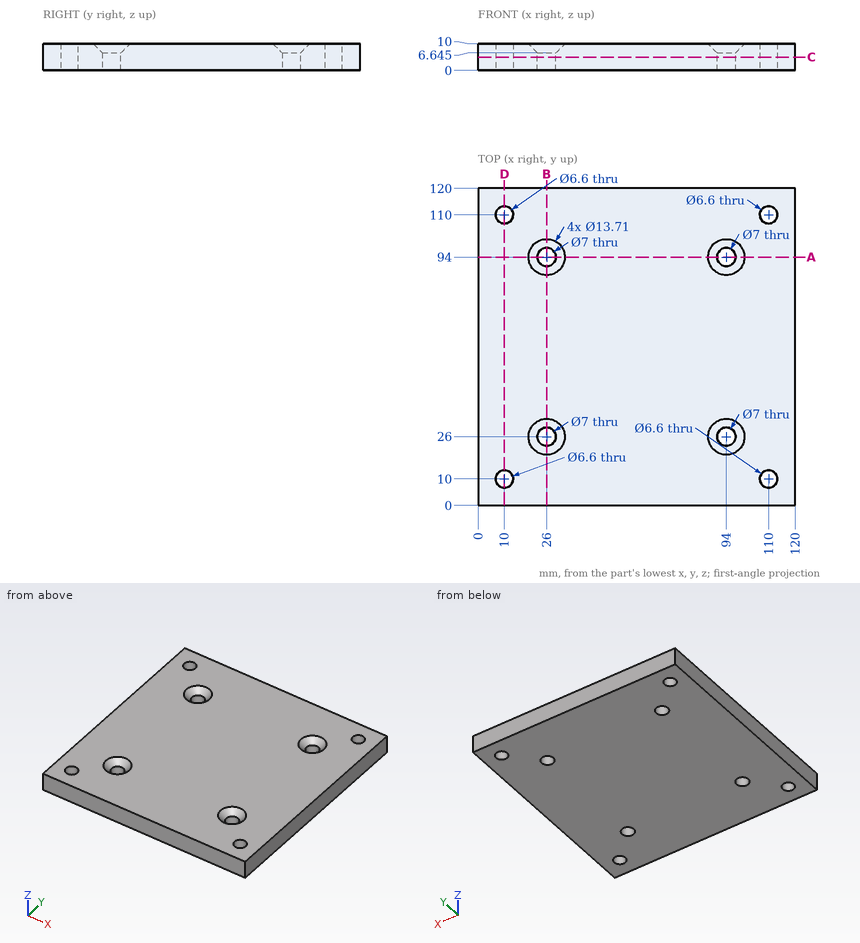
The drawing under review shows one solid part. Ordinate dimensions are in mm from its lowest x, y, z. Coordinates: 2 decimals unless noted, no trailing zeros. Write each loop counter-clockwise with the first axis right and the second up, starting at its lowest first coordinate (ties: lowest second). Pieces come first, ordered by that corner, then holes. Notation, with made-up numbers: (75.25, 30) - (92.25, 30) arc R17 cw to (92.25, 60) - close; hole circle Ø5 at (71, 23). An arc over 180 degrees is marked (long way). Answer in a Markdown table with one row per item. Add a question column.
Q1. We need section D-D, the plane x = 10. State the section outline as (y, z) points, and give its area (3 significant figures).
Q2. For P1, Ø5, axis at y = 58.5, z = 8.5, coming from the -X side, flat-tipped, find the tip position at first contact; note if it passes through.
Q3. For probe 1 along Y at (x, z) = (94, 2); probe 2 along X at (y, z) = (110, 6.25), list the stretches that pass through material, from the lowest coordinate up.
Q4. We need section C-C, the plane z = 5. Count the separate pieces of the cut face and the enclosed holes in it, and give its area (3 significant figures).
Q5. We need section A-A, the plane y = 94. State the section outline as (x, z) points (3 decimals).
Answer list:
| question | item | result |
|---|---|---|
| 1 | outline | (0, 0) - (6.7, 0) - (6.7, 10) - (0, 10) - close; (13.3, 0) - (106.7, 0) - (106.7, 10) - (13.3, 10) - close; (113.3, 0) - (120, 0) - (120, 10) - (113.3, 10) - close |
| 1 | area | 1,070 mm2 |
| 2 | P1 | stops at x = 0 |
| 3 | probe 1 | y = 0 to 22.5, 29.5 to 90.5, 97.5 to 120 |
| 3 | probe 2 | x = 0 to 6.7, 13.3 to 106.7, 113.3 to 120 |
| 4 | separate pieces | 1 |
| 4 | enclosed holes | 8 |
| 4 | area | 14,100 mm2 |
| 5 | outline | (0, 0) - (22.5, 0) - (22.5, 6.645) - (19.145, 10) - (0, 10) - close; (29.5, 0) - (90.5, 0) - (90.5, 6.645) - (87.145, 10) - (32.855, 10) - (29.5, 6.645) - close; (97.5, 0) - (120, 0) - (120, 10) - (100.855, 10) - (97.5, 6.645) - close |
